from build123d import *

# Parameters (mm, degrees)
SKETCH3_W               = 6
SKETCH3_H               = 4
BOSS_EXTRUDE4_DEPTH     = 1
CUT_EXTRUDE2_DEPTH      = 3.5
CUT_EXTRUDE2_DEPTH_BACK = 3.5
SKETCH6_R               = 1.5
CUT_EXTRUDE3_DEPTH      = 18
SKETCH7_OUTSIDE_W       = 11.904
SKETCH7_OUTSIDE_H       = 10.486
SKETCH7_OUTSIDE_R       = 3
CUT_EXTRUDE4_DEPTH      = 10.0000001
CUT_EXTRUDE4_DEPTH_BACK = 10.0000001


with BuildPart() as part:
    # Sketch1 → Revolve5 (revolve)
    with BuildSketch(Plane.XY):
        Polygon((0, 9), (-2.5, 9), (-2.5, 8.5), (-2, 8.5), (-2, 0.5), (-2.25, 0.5), (-2.25, -0.5), (-2, -0.5), (-2, -8.5), (-2.5, -8.5), (-2.5, -9), (0, -9), align=None)
    revolve(axis=Axis((0, 9, 0), (0, -1, 0)))

    # Sketch3 → Boss-Extrude4 (add, symmetric)
    with BuildSketch(Plane.XY):
        Rectangle(SKETCH3_W, SKETCH3_H)
    extrude(amount=BOSS_EXTRUDE4_DEPTH, both=True)

    # Sketch5 → Cut-Extrude2 (cut, two sides)
    with BuildSketch(Plane.XY) as cut_extrude2_sk:
        with BuildLine():
            Line((-1, 9), (-1, 6))
            ThreePointArc((-1, 6), (0, 5), (1, 6))
            Line((1, 6), (1, 9))
            Line((1, 9), (-1, 9))
        make_face()
        with BuildLine():
            Line((-1, -9), (-1, -6))
            ThreePointArc((-1, -6), (0, -5), (1, -6))
            Line((1, -6), (1, -9))
            Line((1, -9), (-1, -9))
        make_face()
    extrude(amount=CUT_EXTRUDE2_DEPTH, mode=Mode.SUBTRACT)
    extrude(cut_extrude2_sk.sketch, amount=-CUT_EXTRUDE2_DEPTH_BACK, mode=Mode.SUBTRACT)

    # Sketch6 → Cut-Extrude3 (cut)
    with BuildSketch(Plane(origin=(0, 9, 0), x_dir=(1, 0, 0), z_dir=(0, 1, 0))):
        Circle(SKETCH6_R)
    extrude(amount=-CUT_EXTRUDE3_DEPTH, mode=Mode.SUBTRACT)

    # Sketch7 outside → Cut-Extrude4 (cut, two sides)
    with BuildSketch(Plane(origin=(0, 0, 0), x_dir=(1, 0, 0), z_dir=(0, 1, 0))) as cut_extrude4_sk:
        Rectangle(SKETCH7_OUTSIDE_W, SKETCH7_OUTSIDE_H)
        Circle(SKETCH7_OUTSIDE_R, mode=Mode.SUBTRACT)
    extrude(amount=CUT_EXTRUDE4_DEPTH, mode=Mode.SUBTRACT)
    extrude(cut_extrude4_sk.sketch, amount=-CUT_EXTRUDE4_DEPTH_BACK, mode=Mode.SUBTRACT)


solid = part.part
Can you work these out from the model? Positions are in its coordinate system, mm. A direction names the side the tool comes from. Give positions to 0.01 mm unless a question says otherwise; leave off trailing zeros. Order: outer loops, then holes, each group sorted by start corner. A loop starts at its lowest first (then second) coordinate and runs counter-clockwise, first axis right, second up. Notation, with made-up numbers: (86, 62.25) - (116, 62.25) arc R8 cw to (116, 71.25) - close; hole circle Ø8 at (88, 49). An arc over 180 degrees is marked (long way). Write each question's results on one line, items separated by ' | '.
1) Suppose I cut it at B-B, the plane z = 0. Write out the boundary of the cut face in (x, y).
Final values:
outline: (-3, -2) - (-2, -2) - (-2, -8.5) - (-2.5, -8.5) - (-2.5, -9) - (-1.5, -9) - (-1.5, 9) - (-2.5, 9) - (-2.5, 8.5) - (-2, 8.5) - (-2, 2) - (-3, 2) - close; (1.5, -9) - (2.5, -9) - (2.5, -8.5) - (2, -8.5) - (2, -2) - (3, -2) - (3, 2) - (2, 2) - (2, 8.5) - (2.5, 8.5) - (2.5, 9) - (1.5, 9) - close
2) I'm going to push flat-ended pins straight in: pin 1 Ø0.9 at (x, y) = (2.5, 0.5) entering from -Z; pin 2 Ø2 at (x, y) = (1.5, 5) entering from -Z; pin 3 Ø1.3 at (y, z) = (7.5, 1.5) entering from +X. Where does each tip first touch, or does it pass through?
Final values:
pin 1: stops at z = -1 | pin 2: stops at z = -1.94 | pin 3: stops at x = 1.81
3) If we mould it in two halves opening along Z, with no side actions, what happens to faces 1 (the face through (2.2, -8.5, 0.2)), 2 (the face through (1.474, -4.556, -1.352)), 3 (the face through (-1.5, 0.13, -0.07))? For each: pulls with the +Z half, pulls with the -Z half, needs draft (parallel to the pull), parting line crosses it, or undercut.
Final values:
face 1: needs draft | face 2: parting line crosses it | face 3: undercut
4) Suppose I cut it at A-A, the plane y = 7. Write out the boundary of the cut face in (x, z), then the cut area to 3 significant figures.
Final values:
outline: (-1, -1.73) - (-1, -1.12) arc R1.5 cw to (-1, 1.12) - (-1, 1.73) arc R2 ccw to start; (1, -1.73) arc R2 ccw to (1, 1.73) - (1, 1.12) arc R1.5 cw to (1, -1.12) - close | area: 3.36 mm^2
5) On a 3-axis mill with a long thin cutter (end or side, diameter ignored), from which of +Z, -Z, +X, -X, +Y, -Y can I reach the whole of each face in a straight line? I mean faces 4 (the face through (2.5, 8.7, 0)), 5 (the face through (0.03, -0.01, 2.25)), 6 (the face through (-2.5, 8.7, 0)). Say none if no direction works.
Final values:
face 4: +X, +Y | face 5: +Z | face 6: -X, +Y
6) Please list where these lines run through material, in increasing order: line 1 along Z through (x, y) = (0, -0.25); line 2 along Y through (x, z) = (-2.35, 0); line 3 along X through (y, z) = (0.75, 0). Write a range as [from, to].
Final values:
line 1: z = [-2.25, -1.5], [1.5, 2.25] | line 2: y = [-9, -8.5], [-2, 2], [8.5, 9] | line 3: x = [-3, -1.5], [1.5, 3]
7) Suppose I cut it at C-C, the plane x = 0. Write out the boundary of the cut face in (y, z).
Final values:
outline: (-5, -2) - (-0.5, -2) - (-0.5, -2.25) - (0.5, -2.25) - (0.5, -2) - (5, -2) - (5, -1.5) - (-5, -1.5) - close; (-5, 1.5) - (5, 1.5) - (5, 2) - (0.5, 2) - (0.5, 2.25) - (-0.5, 2.25) - (-0.5, 2) - (-5, 2) - close
8) Suppose I cut it at D-D, the plane y = 1.75. Write out the boundary of the cut face in (x, z).
Final values:
outline: (-2.83, -1) - (-1.73, -1) arc R2 ccw to (1.73, -1) - (2.83, -1) arc R3 ccw to (2.83, 1) - (1.73, 1) arc R2 ccw to (-1.73, 1) - (-2.83, 1) arc R3 ccw to start; hole circle Ø3 at (0, 0)
